Source: CAD feature listing. Evaluate the final solid. Frame: model axes, mm. Face numbers are marked on the shaded views. A direction names the side the tool comes from. Give positions to 0.01 mm unless a question says otherwise; leave off trailing zeros. Loops run counter-clockwise (first coordinate to the right, second up) from the corner with the lowest first, then second, coordinate; pieces in that order, holes last. Notation, with made-up numbers: M 69,-22 L 82,-22 A30 cw 82,6 Z; hole C -5,39 d9. An arc over 180 degrees is marked long. Put each result on its own line as item: value. Start each with the question number.
Autodesk Inventor part; units mm, degrees
ref_plane "YZ Plane" through (0, 0, 0) normal (1, 0, 0) x (0, 1, 0)
ref_plane "XZ Plane" through (0, 0, 0) normal (0, 1, 0) x (-1, 0, 0)
ref_plane "XY Plane" through (0, 0, 0) normal (0, 0, 1) x (1, 0, 0)
sketch "Sketch1" plane through (0, 0, 0) normal (0, 0, 1) x (1, 0, 0)
  arc A0 (0, 990) -> (-990, 0) centre (0, 0) ccw
  arc A1 (0, 980) -> (-980, 0) centre (0, 0) ccw
  line L0 (-990, 0) -> (-980, 0)
  line L1 (0, 990) -> (0, 980)
  line L2 (0, -214.865) -> (0, 1289.19)
  dimension "d0" = 10
  dimension "d1" = 990
  dimension "d2" = 0
  dimension "d3" = 0
revolve "Revolution1" add sketch "Sketch1" angle 90 about axis through (0, -10, 0) along (0, 1, 0)
sketch "Sketch2" plane through (0, 0, 0) normal (1, 0, 0) x (0, -0.7071068, -0.7071068)
  arc A0 (-700.0357, 700.0357) -> (-700.0357, -700.0357) centre (0, 0) ccw
  arc A1 (-692.9646, 692.9646) -> (-692.9646, -692.9646) centre (0, 0) ccw
  line L0 (-692.9646, 692.9646) -> (-700.0357, 700.0357)
  line L1 (-700.0357, -700.0357) -> (-692.9646, -692.9646)
extrude "Extrusion2" add sketch "Sketch2" along normal blind 900
equation "\"d0\" = thickness"
equation "\"thickness\" = 10"
equation "\"hoop_angle_z\" = 45deg"
equation "\"hoop_bearing_length\" = 5deg"
equation "\"hoop_cable_diam\" = 5"
equation "\"hoop_cable_pulley_diam\" = 22"
equation "\"rack_tooth_addendum\" = 5"
equation "\"rack_tooth_dedendum\" = 5"
equation "\"rack_tooth_thickness\" = 5"
equation "\"secure_arm_angle\" = 20deg"
equation "\"secure_arm_hold_length\" = 35"
equation "\"secure_arm_radii\" = 9"
equation "\"support_baseClamp_platformLengthBuffer\" = 35"
equation "\"support_baseClamp_platformThickness\" = 15"
equation "\"support_baseClamp_platformWidthBuffer\" = 0"
equation "\"support_baseClamp_sleeveHoleDiameter\" = 12"
equation "\"support_baseClamp_sleeveSweepTerminationAngle\" = 55deg"
equation "\"support_baseClamp_thickness\" = 8"
equation "\"support_frame_endHoleBuffer\" = 25"
equation "\"support_frame_squareBarFillet\" = 2"
equation "\"support_frame_squareBarThickness\" = 5"
equation "\"hoop_tabs_thickness\" = 6"
equation "\"hoop_tabs_hole\" = 4"
equation "\"wheelchair_deployed_width\" = 635"
equation "\"wheelchair_deployed_length\" = 1067"
equation "\"wheelchair_deployed_height\" = 914"
properties part number "cover2_sule_inner"
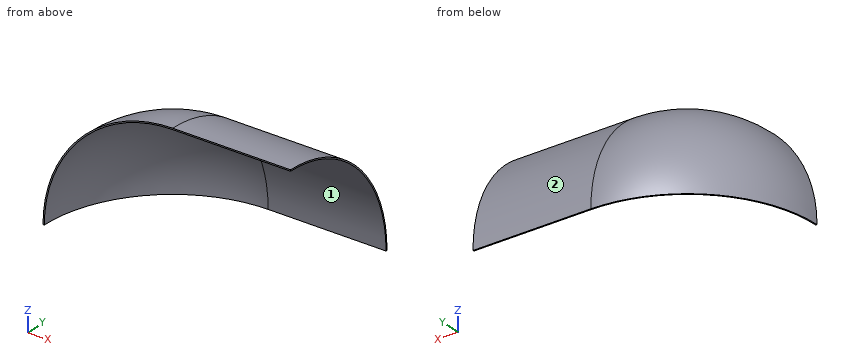
1. Section D-D, the plane x = -87. Output: boundary loops of the cut face in (y, z).
2. Contact query for flat-ended pins moving along their axis: pin 1 (8 mm diameter, centred on x = -390.5, z = 728, fed in from -Y); pin 2 (3 mm diameter, centred on x = 647, z = 566, fed in from +Y); pin 3 (12 mm diameter, centred on x = 559, z = 180.5, fed in from +Y). Output: stop coordinate, or through.
3. Section A-A, the plane z = 682. Output: boundary loops of the cut face in (x, y).
4. Section C-C, the plane x = 590.5. Output: boundary loops of the cut face in (y, z).
5. Set-up query: the marked faces 1 and 2. Return all of +Z, -Z, +X, -X, +Y, -Y with unobstructed straight access to the full face (end or side cutting, diameter ignored); none if empty.
6. Section B-B, the plane y = 400.5. Output: boundary loops of the cut face in (x, z), plus the area to 3 significant figures.
7. Ray query, line 1 (Z direction, x = 764, y = 559.5); line 2 (Z direction, x = 288, y = 104.5); line 3 (X direction, y = 220.5, z = 54.5) (3 decimals). Return the intervals inside material, ascending.
Results found:
1. outline: M 0,976.13 A976.13 cw 976.13,0 L 986.17,0 A986.17 ccw 0,986.17 Z
2. pin 1: y = 520.87
2. pin 2: y = 813.29
2. pin 3: y = 974.5
3. outline: M -717.62,0 L -703.76,0 A703.76 cw 0,703.76 L 900,703.76 L 900,717.62 L 0,717.62 A717.62 ccw Z
4. outline: M 0,980 A980 cw 980,0 L 990,0 A990 ccw 0,990 Z
5. face 1: -Z, +X, -Y
5. face 2: +Z, +X, -X, +Y
6. outline: M -905.37,0 L -894.43,0 A894.43 cw 0,894.43 L 900,894.43 L 900,905.37 L 0,905.37 A905.37 ccw Z
6. area: 25,300 mm²
7. line 1: 804.59 to 816.74
7. line 2: 974.41 to 984.47
7. line 3: -963.592 to -953.315
